Input: part model. Units: mm. Frame: model coordinates. Give positions to 0.01 mm unless a question says otherwise; leave off trailing zeros. Loops run counter-clockwise (first coordinate to the right, second up) from the corner with the lowest first, then second, coordinate; pieces in that order, holes last. Notation, with made-up numbers: (-24.5, 8) - (31.5, 8) arc R26 cw to (31.5, 26) - close; hole circle Ø1 at (-28.75, 34.5). An arc over 180 degrees is marked (long way). One line per question, with ' | ' between items. Start each with the question number.
from build123d import *

# Parameters (mm, degrees)
F0_W     = 500
F0_H     = 430
F1_DEPTH = 1500
F3_DEPTH = 430
F4_R     = 125
F5_DEPTH = 500
F6_R     = 160
F7_DEPTH = 500


with BuildPart() as f1:
    # F0 (on Front) → F1 (new body)
    with BuildSketch(Plane.XZ):
        Rectangle(F0_W, F0_H)
    extrude(amount=-F1_DEPTH)

    # F2 (on face) → F3 (join)
    with BuildSketch(Plane.XY.offset(215)):
        with BuildLine():
            Line((-250, 1500), (250, 1500))
            ThreePointArc((250, 1500), (0, 1750), (-250, 1500))
        make_face()
    extrude(amount=-F3_DEPTH)

    # F4 (on face) → F5 (cut)
    with BuildSketch(Plane.XY.offset(215)):
        with Locations((0, 1505)):
            Circle(F4_R)
    extrude(amount=-F5_DEPTH, mode=Mode.SUBTRACT)

    # F6 (on face) → F7 (cut)
    with BuildSketch(Plane.XY.offset(215)):
        with Locations((0, 250)):
            Circle(F6_R)
    extrude(amount=-F7_DEPTH, mode=Mode.SUBTRACT)


solid = f1.part
Q1. Line query: L1, parallel to Y at x = 0, z = 65; L2, parallel to Y at x = -4, z = 156.5; L3, parallel to X at y = 281.5, z = -90.5. Output: solid intervals per line, ascending. Write a range as from..to.
Q2. Section B-B, the plane x = -83.5. Output: boundary loops of the cut face in (y, z), plus the area to 3 significant figures.
Q3. First-contact query: pin 1 (3 mm diameter, centred on y = 1530, z = 103.5, fed in from +X); pin 2 (12 mm diameter, centred on x = 186, z = 76.5, fed in from +Y). Flat tips, straight axial feed; report the tip coordinate or a pass-through.
Q4. Section C-C, the plane z = 65. Output: boundary loops of the cut face in (x, y), plus the area to 3 significant figures.
Q5. Section A-A, the plane y = 250. Output: boundary loops of the cut face in (x, z), plus the area to 3 significant figures.
Q6. Draft query along X for faces 1 (the face through (-250, 740, -3)), 2 (the face through (-16.273, 1628.936, 3.01)), 3 (the face through (250, 740, -3)). Return one class per face: +X half, -X half, draft (parallel to the pull), parting line (faces both ways), or undercut.
Q7. Section D-D, the plane x = 0. Output: boundary loops of the cut face in (y, z), plus the area to 3 significant figures.
Solved:
1) L1: y = 0..90, 410..1380, 1630..1750 | L2: y = 0..90.05, 409.95..1380.06, 1629.94..1749.97 | L3: x = -250..-156.87, 156.87..250
2) outline: (0, -215) - (113.52, -215) - (113.52, 215) - (0, 215) - close; (386.48, -215) - (1411.98, -215) - (1411.98, 215) - (386.48, 215) - close; (1598.02, -215) - (1735.64, -215) - (1735.64, 215) - (1598.02, 215) - close | area: 549,000 mm²
3) pin 1: stops at x = 248.37 | pin 2: stops at y = 1673.49
4) outline: (-250, 0) - (250, 0) - (250, 1500) arc R250 ccw to (-250, 1500) - close; hole circle Ø320 at (0, 250); hole circle Ø250 at (0, 1505) | area: 719,000 mm²
5) outline: (-250, -215) - (-160, -215) - (-160, 215) - (-250, 215) - close; (160, -215) - (250, -215) - (250, 215) - (160, 215) - close | area: 77,400 mm²
6) face 1: -X half | face 2: undercut | face 3: +X half
7) outline: (0, -215) - (90, -215) - (90, 215) - (0, 215) - close; (410, -215) - (1380, -215) - (1380, 215) - (410, 215) - close; (1630, -215) - (1750, -215) - (1750, 215) - (1630, 215) - close | area: 507,000 mm²
